Can you work these out from the model? Positions are in its coordinate system, mm. A direction names the side the tool comes from. Give positions to 0.01 mm unless a question says otherwise; leave off trailing zeros. Order: outer loops, then holes, each group sorted by start corner. A loop starts at its lowest first (then second) coordinate and runs counter-clockwise, first axis right, second up. Notation, with made-up numbers: (18, 11.25) - (39, 11.25) arc R7 cw to (39, 24.25) - close; hole circle Ø10 at (-5.5, 70). An arc over 180 degrees is marked (long way). One line per question, with ' | ' between items.
```python
from build123d import *

# Parameters (mm, degrees)
SKETCH2_R           = 62.854
SKETCH2_R_2         = 61.838
BOSS_EXTRUDE1_DEPTH = 105.5
SKETCH3_R           = 10.7
CUT_EXTRUDE1_DEPTH  = 105.5
SKETCH4_R           = 10.65
CUT_EXTRUDE2_DEPTH  = 105.5
SKETCH5_R           = 10.65
CUT_EXTRUDE3_DEPTH  = 105.5


with BuildPart() as part:
    # Sketch2 → Boss-Extrude1 (new body)
    with BuildSketch(Plane(origin=(0, 0, 0), x_dir=(-1, 0, 0), z_dir=(0, 1, 0))):
        with Locations(Location((4.078625789, 4.753613482, 0), (0, 0, 270))):
            Circle(SKETCH2_R)
        with Locations(Location((4.078625789, 4.753613482, 0), (0, 0, 270))):
            Circle(SKETCH2_R_2, mode=Mode.SUBTRACT)
    extrude(amount=BOSS_EXTRUDE1_DEPTH)

    # Sketch3 → Cut-Extrude1 (cut)
    with BuildSketch(Plane(origin=(-8.080908151, 23.599932993, 4.753613482), x_dir=(-1, 0, 0), z_dir=(0, 0, -1))):
        with Locations(Location((-4.002282363, 7.900067007, 0), (0, 0, 90))):
            Circle(SKETCH3_R)
    extrude(amount=-CUT_EXTRUDE1_DEPTH, mode=Mode.SUBTRACT)

    # Sketch4 → Cut-Extrude2 (cut)
    with BuildSketch(Plane(origin=(-4.078625789, 23.599932993, 9.571680039), x_dir=(0, 0, -1), z_dir=(1, 0, 0))):
        with Locations(Location((4.818066557, 10.350067007, 0), (0, 0, 270))):
            Circle(SKETCH4_R)
    extrude(amount=CUT_EXTRUDE2_DEPTH, mode=Mode.SUBTRACT)

    # Sketch5 → Cut-Extrude3 (cut)
    with BuildSketch(Plane(origin=(-4.078625789, 23.599932993, 9.571680039), x_dir=(0, 0, -1), z_dir=(1, 0, 0))):
        with Locations(Location((4.818066557, 58.750067007, 0), (0, 0, 90))):
            Circle(SKETCH5_R)
    extrude(amount=-CUT_EXTRUDE3_DEPTH, mode=Mode.SUBTRACT)


solid = part.part
```
(1) Will these pins go through, and if not, where does the flat tip stop? pin 1 (5 mm diameter, centred on x = -35, z = -45, fed in from +Y); pin 2 (5 mm diameter, centred on x = 0.5, y = 86.5, fed in from +Z); pin 3 (6 mm diameter, centred on x = -27.5, y = 11.5, fed in from +Z); pin 4 (13 mm diameter, centred on y = 33.95, z = 4.75, fed in from -X).
Answer below:
pin 1: through | pin 2: z = 67.57 | pin 3: z = 64.2 | pin 4: x = -66.93
(2) Imagine slicing it at C-C (x = 2.5). List the corners of the cut face in (y, z) for me, and give its area (3 significant figures).
Answer below:
outline: (0, -57.76) - (105.5, -57.76) - (105.5, -56.73) - (0, -56.73) - close; (0, 66.24) - (23.06, 66.24) - (23.06, 67.26) - (0, 67.26) - close; (39.94, 66.24) - (105.5, 66.24) - (105.5, 67.26) - (39.94, 67.26) - close | area: 198 mm^2
(3) If I drill on line 1 (X direction, y = 45.5, z = -51.5); line 2 (Z direction, x = 43, y = 95); line 3 (X direction, y = 77, z = 55), over which ranges is the centre line in solid material (lowest first)?
Answer below:
line 1: -32.12 to -29.76, 21.6 to 23.96 | line 2: -36.89 to -35.34, 44.85 to 46.4 | line 3: -41.84 to -40.12, 31.97 to 33.68
(4) On a 3-axis mill with a long thin cutter (end or side, diameter ignored), from which of +Z, -Z, +X, -X, +Y, -Y can I reach the whole of each face in a straight line? I mean faces 1 (the face through (19.606, 52.012, -52.369)), 2 (the face through (3.15, 23.61, 66.62)), 3 (the face through (57.792, 41.799, -2.444)). Say none if no direction works.
Answer below:
face 1: +Y, -Y | face 2: +Z | face 3: +X
(5) Imagine slicing it at A-A (x = -41.5). List the corners of the cut face in (y, z) for me.
Answer below:
outline: (0, -45.75) - (105.5, -45.75) - (105.5, -44.48) - (0, -44.48) - close; (0, 53.98) - (105.5, 53.98) - (105.5, 55.25) - (0, 55.25) - close
(6) If we mould it in two halves opening along Y, with no side actions, what happens to faces 4 (the face through (37.5, 0, -41.5)), 5 (the face through (37.5, 105.5, -41.5)), 6 (the face through (-65.95, 74.5, 11.95))? For each: released by +Y, released by -Y, zero draft, split by the parting line, or undercut.
Answer below:
face 4: released by -Y | face 5: released by +Y | face 6: undercut
(7) Imagine slicing it at D-D (y = 52.5). List the corners of the cut face in (x, z) for me, and give its area (3 significant figures).
Answer below:
outline: circle Ø125.71 at (-4.08, 4.75); hole circle Ø123.68 at (-4.08, 4.75) | area: 398 mm^2
